Can you work these out from the drawing? Everything is in mm from the part's minimum corner. A direction names the side the tool comes from. Give positions to 0.01 mm unless a question says otherwise; leave off trailing zeros. Write each loop counter-clockwise with the first axis right and the second up, starting at its lowest first coordinate (ties: lowest second). Pieces come first, ordered by that corner, then holes. Notation, with made-up numbers: (30, -21.5) - (87, -21.5) arc R7 ccw to (87, -10.5) - close; hole circle Ø1 at (9.5, -4.5). An arc over 180 degrees is marked (long way). Use a Markdown table: item, result.
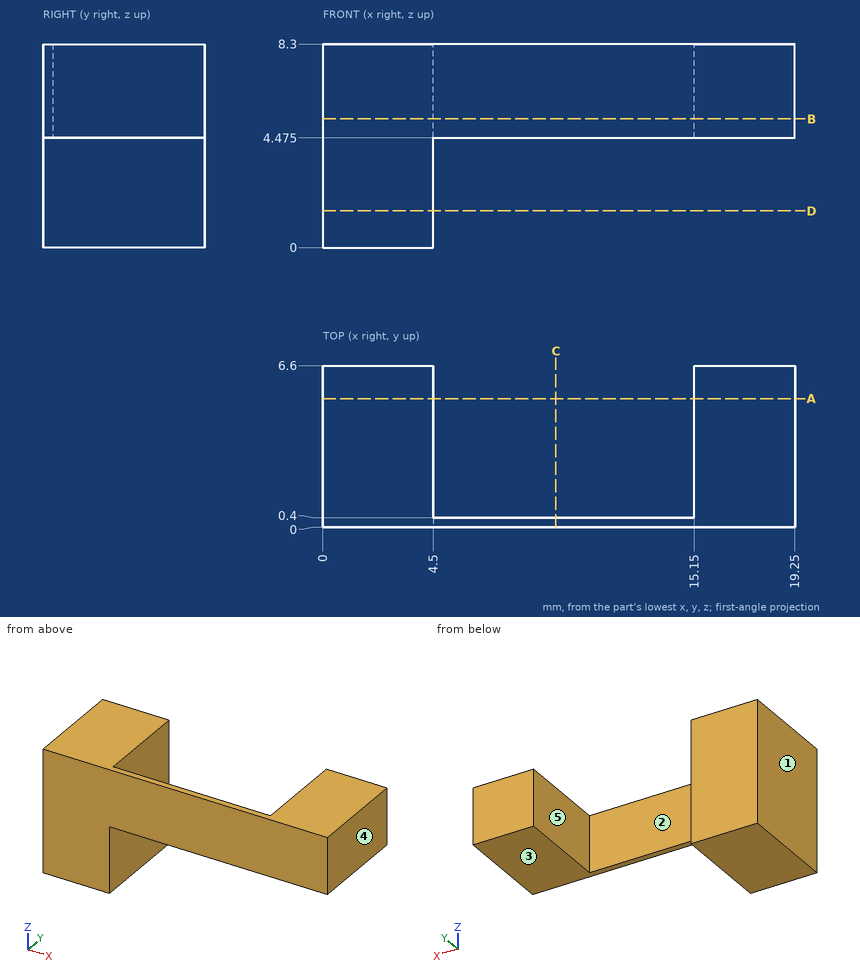
Item 1: If we section it at C-C, the plane x = 9.5: Write out the boundary of the cut face in (y, z) (3 decimals).
Values:
| item | result |
|---|---|
| outline | (0, 4.475) - (0.4, 4.475) - (0.4, 8.3) - (0, 8.3) - close |
Item 2: Will these pins go through, and if not, where does the flat tip stop? pin 1 Ø2 at (x, z) = (16.5, 2.5) entering from +Y; pin 2 Ø2 at (x, y) = (16, 4.5) entering from -Z (3 decimals); pin 3 Ø4 at (x, z) = (11, 5.5) entering from +Y.
Values:
| item | result |
|---|---|
| pin 1 | passes through |
| pin 2 | stops at z = 4.475 |
| pin 3 | stops at y = 0.4 |
Item 3: If we section it at B-B, the plane z = 5.25: Write out the boundary of the cut face in (x, y).
Values:
| item | result |
|---|---|
| outline | (0, 0) - (19.25, 0) - (19.25, 6.6) - (15.15, 6.6) - (15.15, 0.4) - (4.5, 0.4) - (4.5, 6.6) - (0, 6.6) - close |
Item 4: If we section it at A-A, the plane y = 5.25: Write out the boundary of the cut face in (x, z) (3 decimals), plus the area to 3 significant figures.
Values:
| item | result |
|---|---|
| outline | (0, 0) - (4.5, 0) - (4.5, 8.3) - (0, 8.3) - close; (15.15, 4.475) - (19.25, 4.475) - (19.25, 8.3) - (15.15, 8.3) - close |
| area | 53.0 mm2 |
Item 5: If we section it at D-D, the plane z = 1.5: Write out the boundary of the cut face in (x, y), plus the area to 3 significant figures.
Values:
| item | result |
|---|---|
| outline | (0, 0) - (4.5, 0) - (4.5, 6.6) - (0, 6.6) - close |
| area | 29.7 mm2 |
Item 6: Thinking about a two-plate mould opening in X: for the marked faces 1, 2 and 3, which applies, +X half, -X half, draft (parallel to the pull), parting line (faces both ways), or undercut?
Values:
| item | result |
|---|---|
| face 1 | -X half |
| face 2 | undercut |
| face 3 | draft |
Item 7: I need wall thicknesses on line 1 along X through (y, z) = (4.25, 5.5); line 2 along Y through (x, z) = (5.25, 5.75); line 3 along X through (y, z) = (2, 3.5). Which ranges of each line are inside material? Lowest first, please. Write a range as [from, to].
Values:
| item | result |
|---|---|
| line 1 | x = [0, 4.5], [15.15, 19.25] |
| line 2 | y = [0, 0.4] |
| line 3 | x = [0, 4.5] |
Item 8: For the marked faces 4 and 5, which set-ups out of +Z, -Z, +X, -X, +Y, -Y let a thin tool reach every point of the face, with its end or its side?
Values:
| item | result |
|---|---|
| face 4 | +Z, -Z, +X, +Y, -Y |
| face 5 | +Z, -Z, +Y |
